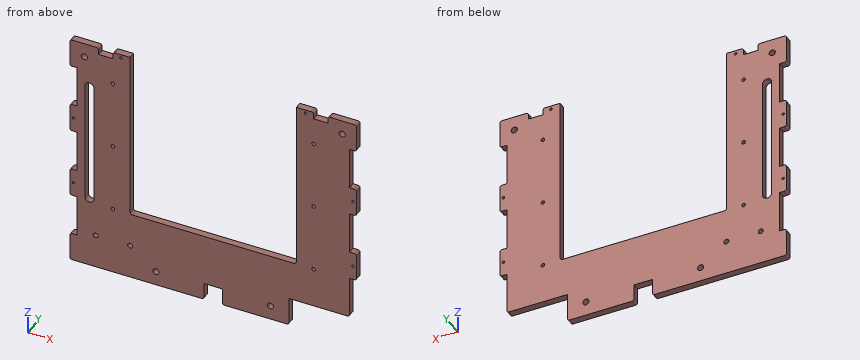
Autodesk Inventor part; units mm, degrees
ref_plane "YZ Plane" through (0, 0, 0) normal (1, 0, 0) x (0, 1, 0)
ref_plane "XZ Plane" through (0, 0, 0) normal (0, 1, 0) x (-1, 0, 0)
ref_plane "XY Plane" through (0, 0, 0) normal (0, 0, 1) x (1, 0, 0)
sketch "Sketch1" plane through (0, 0, 0) normal (0, 1, 0) x (-1, 0, 0)
  line L0 (125, -92.5) -> (-125, -92.5)
  line L1 (-125, -92.5) -> (-125, 92.5)
  line L2 (-125, 92.5) -> (125, 92.5)
  line L3 (125, 92.5) -> (125, -92.5)
  line L4 (125, -92.5) -> (-125, 92.5) construction
  line L5 (-125, -92.5) -> (125, 92.5) construction
  line L6 (72.5, -57.5) -> (-72.5, -57.5)
  line L7 (-72.5, -57.5) -> (-72.5, 57.5)
  line L8 (-72.5, 57.5) -> (72.5, 57.5)
  line L9 (72.5, 57.5) -> (72.5, -57.5)
  line L10 (72.5, -57.5) -> (-72.5, 57.5) construction
  line L11 (-72.5, -57.5) -> (72.5, 57.5) construction
  line L12 (-90.9745, -29.5734) -> (-84.0255, -29.5734) construction
  line L13 (-84.0255, -29.5734) -> (-84.0255, 29.5734) construction
  line L14 (-84.0255, 29.5734) -> (-90.9745, 29.5734) construction
  line L15 (-90.9745, 29.5734) -> (-90.9745, -29.5734) construction
  line L16 (-90.9745, -29.5734) -> (-84.0255, 29.5734) construction
  line L17 (-84.0255, -29.5734) -> (-90.9745, 29.5734) construction
  line L18 (81.5853, -29.5734) -> (93.4147, -29.5734) construction
  line L19 (93.4147, -29.5734) -> (93.4147, 29.5734) construction
  line L20 (93.4147, 29.5734) -> (81.5853, 29.5734) construction
  line L21 (81.5853, 29.5734) -> (81.5853, -29.5734) construction
  line L22 (81.5853, -29.5734) -> (93.4147, 29.5734) construction
  line L23 (93.4147, -29.5734) -> (81.5853, 29.5734) construction
  point P0 (0, 0)
  point P1 (-87.5, 0)
  point P2 (87.5, 0)
  dimension "d0" = 175
  dimension "d1" = 87.5
  dimension "d2" = 145
  dimension "d4" = 185
  dimension "d5" = 250
  dimension "d15" = 35
extrude "Extrusion1" add sketch "Sketch1" along normal blind 6
sketch "Sketch2" plane through (0, 6, 0) normal (0, 1, 0) x (1, 0, 0)
  line L0 (72.5, -57.5) -> (-72.5, -57.5)
  line L1 (-125, -92.5) -> (125, -92.5)
  line L2 (-72.5, -57.5) -> (72.5, -57.5)
  line L3 (72.5, -57.5) -> (72.5, -92.5)
  line L4 (72.5, -92.5) -> (-72.5, -92.5)
  line L5 (-72.5, -92.5) -> (-72.5, -57.5)
  point P0 (0, 0)
extrude "Extrusion2" cut sketch "Sketch2" against normal through all
sketch "Sketch3" plane through (0, 0, 0) normal (0, -1, 0) x (1, 0, 0)
  line L0 (-125, 92.5) -> (-125, -92.5)
  line L1 (-125, -92.5) -> (125, -92.5)
  line L2 (125, -92.5) -> (125, 92.5)
  line L3 (-125, -117.5) -> (66, -117.5)
  line L4 (66, -117.5) -> (66, -92.5)
  line L5 (66, -92.5) -> (-125, -92.5)
  line L6 (-125, -92.5) -> (-125, -117.5)
  line L7 (-125, -117.5) -> (66, -92.5) construction
  line L8 (66, -117.5) -> (-125, -92.5) construction
  point P0 (0, 0)
  point P1 (-29.5, -105)
  dimension "d10" = 59
  dimension "d11" = 25
extrude "Extrusion3" add sketch "Sketch3" against normal blind 6
sketch "Sketch4" plane through (0, 6, 0) normal (0, 1, 0) x (1, 0, 0)
  line L0 (-72.5, -92.5) -> (-72.5, 57.5)
  line L1 (-72.5, 57.5) -> (72.5, 57.5)
  line L2 (-125, -92.5) -> (-72.5, -92.5)
  line L3 (-108, 53.5) -> (-108, -52.5) construction
  line L4 (-112, 53.5) -> (-112, -52.5)
  line L5 (-104, -52.5) -> (-104, 53.5)
  arc A0 (-104, 53.5) -> (-112, 53.5) centre (-108, 53.5) ccw
  arc A1 (-112, -52.5) -> (-104, -52.5) centre (-108, -52.5) ccw
  point P0 (0, 0)
  point P1 (-108, 0.5)
  dimension "d16" = 8
  dimension "d17" = 108
  dimension "d18" = 40
extrude "Extrusion4" cut sketch "Sketch4" against normal through all
sketch "Sketch5" plane through (0, 0, 0) normal (0, -1, 0) x (1, 0, 0)
  line L0 (125, 92.5) -> (-125, 92.5)
  line L1 (72.5, -57.5) -> (-72.5, -57.5)
  circle A0 centre (-87.5, 62.5) radius 1.6
  circle A1 centre (-87.5, 2.5) radius 1.6
  circle A2 centre (-87.5, -57.5) radius 1.6
  circle A3 centre (87.5, 62.5) radius 1.6
  circle A4 centre (87.5, 2.5) radius 1.6
  circle A5 centre (87.5, -57.5) radius 1.6
  line L2 (87.5, 62.5) -> (-87.5, 62.5) construction
  line L3 (0, -57.5) -> (0, 62.5) construction
  line L4 (-95, -72.5) -> (-80, -72.5) construction
  line L5 (-80, -72.5) -> (-80, 77.5) construction
  line L6 (-80, 77.5) -> (-95, 77.5) construction
  line L7 (-95, 77.5) -> (-95, -72.5) construction
  line L8 (-95, -72.5) -> (-80, 77.5) construction
  line L9 (-80, -72.5) -> (-95, 77.5) construction
  point P0 (-72.5, 92.5)
  point P1 (0, 0)
  dimension "d21" = 60
  dimension "d22" = 60
  dimension "d23" = 175
  dimension "d24" = 3.2
  dimension "d25" = 150
  dimension "d26" = 15
extrude "Extrusion5" cut sketch "Sketch5" against normal through all
sketch "Sketch6" plane through (0, 6, 0) normal (0, 1, 0) x (1, 0, 0)
  circle A0 centre (-87.5, 57.5) radius 1.6
  line L0 (66, 117.5) -> (-125, 117.5)
  line L1 (-112.5, 60.5) -> (-62.5, 60.5) construction
  line L2 (-62.5, 60.5) -> (-62.5, 114.5) construction
  line L3 (-62.5, 114.5) -> (-112.5, 114.5) construction
  line L4 (-112.5, 114.5) -> (-112.5, 60.5) construction
  line L5 (-112.5, 60.5) -> (-62.5, 114.5) construction
  line L6 (-62.5, 60.5) -> (-112.5, 114.5) construction
  circle A1 centre (-102.5, 87.5) radius 2.2
  circle A2 centre (-72.5, 87.5) radius 2.2
  circle A3 centre (-50, 105) radius 2.7
  circle A4 centre (50, 105) radius 2.7
  line L7 (125, -92.5) -> (125, 92.5)
  line L8 (-125, 117.5) -> (-125, -92.5)
  line L9 (-125, -92.5) -> (-72.5, -92.5)
  circle A5 centre (-112.5, -80) radius 2.7
  circle A6 centre (112.5, -80) radius 2.7
  point P0 (0, 0)
  point P1 (-87.5, 87.5)
  dimension "d29" = 50
  dimension "d30" = 54
  dimension "d31" = 3
  dimension "d32" = 4.4
  dimension "d33" = 30
  dimension "d34" = 15
  dimension "d42" = 12.5
  dimension "d43" = 50
  dimension "d44" = 50
  dimension "d45" = 5.4
  dimension "d46" = 12.5
  dimension "d47" = 12.5
  dimension "d48" = 12.5
  dimension "d49" = 5.4
  dimension "d71" = 12.5
extrude "Extrusion6" cut sketch "Sketch6" against normal through all contours A1 | A2 | A3 | A4 | A5 | A6
sketch "Sketch7" plane through (0, 6, 0) normal (0, 1, 0) x (1, 0, 0)
  line L0 (66, 117.5) -> (-125, 117.5)
  line L1 (-8, 102.5) -> (8, 102.5)
  line L2 (8, 102.5) -> (8, 117.5)
  line L3 (8, 117.5) -> (-8, 117.5)
  line L4 (-8, 117.5) -> (-8, 102.5)
  line L5 (-8, 102.5) -> (8, 117.5) construction
  line L6 (8, 102.5) -> (-8, 117.5) construction
  point P0 (0, 0)
  point P1 (0, 110)
  dimension "d38" = 16
  dimension "d39" = 15
extrude "Extrusion7" cut sketch "Sketch7" against normal through all
sketch "Sketch8" plane through (0, 6, 0) normal (0, 1, 0) x (1, 0, 0)
  line L0 (-125, 117.5) -> (-125, -92.5)
  line L1 (72.5, -92.5) -> (125, -92.5)
  line L2 (125, -92.5) -> (125, 92.5)
  line L3 (125, 92.5) -> (66, 92.5)
  line L4 (125, 92.5) -> (118.9, 92.5)
  line L5 (118.9, 92.5) -> (118.9, 55.8333)
  line L6 (118.9, 55.8333) -> (125, 55.8333)
  line L7 (125, 55.8333) -> (125, 92.5)
  line L8 (125, -67.5) -> (118.9, -67.5)
  line L9 (118.9, -67.5) -> (118.9, -30.8333)
  line L10 (118.9, -30.8333) -> (125, -30.8333)
  line L11 (125, -30.8333) -> (125, -67.5)
  line L12 (125, 30.8333) -> (118.9, 30.8333)
  line L13 (118.9, 30.8333) -> (118.9, -5.8333)
  line L14 (118.9, -5.8333) -> (125, -5.8333)
  line L15 (125, -5.8333) -> (125, 30.8333)
  line L16 (-125, 92.5) -> (-118.9, 92.5)
  line L17 (-118.9, 92.5) -> (-118.9, 55.8333)
  line L18 (-118.9, 55.8333) -> (-125, 55.8333)
  line L19 (-125, 55.8333) -> (-125, 92.5)
  line L20 (-125, 30.8333) -> (-118.9, 30.8333)
  line L21 (-118.9, 30.8333) -> (-118.9, -5.8333)
  line L22 (-118.9, -5.8333) -> (-125, -5.8333)
  line L23 (-125, -5.8333) -> (-125, 30.8333)
  line L24 (-125, -67.5) -> (-118.9, -67.5)
  line L25 (-118.9, -67.5) -> (-118.9, -30.8333)
  line L26 (-118.9, -30.8333) -> (-125, -30.8333)
  line L27 (-125, -30.8333) -> (-125, -67.5)
  circle A0 centre (121.95, 43.3333) radius 1.1
  circle A1 centre (121.95, -18.3333) radius 1.1
  circle A2 centre (-121.95, -18.3333) radius 1.1
  circle A3 centre (-121.95, 43.3333) radius 1.1
  line L28 (121.95, 55.8333) -> (121.95, 43.3333) construction
  line L29 (-121.95, 55.8333) -> (-121.95, 43.3333) construction
  point P0 (0, 0)
  dimension "d50" = 25
  dimension "d51" = 6.1
  dimension "d52" = 25
  dimension "d53" = 25
  dimension "d54" = 2.2
  dimension "d55" = 12.5
  dimension "d56" = 12.5
extrude "Extrusion8" cut sketch "Sketch8" against normal through all
sketch "Sketch9" plane through (0, 6, 0) normal (0, 1, 0) x (1, 0, 0)
  circle A0 centre (-121.95, -18.3333) radius 1.1
  line L0 (-118.9, -67.5) -> (-125, -67.5)
  line L1 (-125, -92.5) -> (-72.5, -92.5)
  line L2 (72.5, -92.5) -> (125, -92.5)
  line L3 (-100, -92.5) -> (-87.5, -92.5)
  line L4 (-87.5, -92.5) -> (-87.5, -86.4)
  line L5 (-87.5, -86.4) -> (-100, -86.4)
  line L6 (-100, -86.4) -> (-100, -92.5)
  line L7 (100, -92.5) -> (87.5, -92.5)
  line L8 (87.5, -92.5) -> (87.5, -86.4)
  line L9 (87.5, -86.4) -> (100, -86.4)
  line L10 (100, -86.4) -> (100, -92.5)
  circle A1 centre (-80.5, -89.45) radius 1.1
  circle A2 centre (80.5, -89.45) radius 1.1
  line L11 (-80.5, -89.45) -> (-87.5, -89.45) construction
  line L12 (-125, -67.5) -> (-125, -92.5)
  line L13 (-72.5, -92.5) -> (-72.5, 57.5)
  line L14 (72.5, 57.5) -> (72.5, -92.5)
  line L15 (125, -92.5) -> (125, -67.5)
  point P0 (0, 0)
  dimension "d60" = 12.5
  dimension "d66" = 25
  dimension "d68" = 8
  dimension "d69" = 8
  dimension "d70" = 25
extrude "Extrusion9" cut sketch "Sketch9" against normal through all contours L6 L5 L4 L1 | L8 L9 L10 L2 | A1 | A2
fillet "Fillet1" radius 2 9 edges at (125, 3, 92.5) (72.5, 3, -57.5) (-125, 3, 92.5) (-72.5, 3, -57.5) (66, 3, -117.5) (-125, 3, -117.5) (8, 3, -117.5) (-8, 3, -117.5) (118.9, 3, -92.5)
fillet "Fillet2" radius 2 15 edges at (125, 3, -55.8333) (125, 3, -30.8333) (125, 3, 5.8333) (125, 3, 30.8333) (125, 3, 67.5) (-125, 3, 67.5) (-125, 3, 30.8333) (-125, 3, 5.8333) (-125, 3, -30.8333) (-125, 3, -55.8333) (-125, 3, -92.5) (-100, 3, 92.5) (-87.5, 3, 92.5) (87.5, 3, 92.5) (100, 3, 92.5)
equation "\"d22\" = d21"
equation "\"d53\" = d52"
equation "\"d55\" = 0.5 * d52"
equation "\"d56\" = d55"
properties part number "InnerTop"
Model file for the job. Use its own axes, mm. Round coordinates to 2 decimals unless told otherwise and drop trailing zeros. Order: outer loops, then holes, each group sorted by start corner. A loop starts at its lowest first (then second) coordinate and runs counter-clockwise, first axis right, second up. Notation, with made-up numbers: (56, -5) -> (91, -5) arc R9 cw to (91, -1) -> close; hole circle Ø2 at (-3.5, 5.5). An arc over 180 degrees is marked (long way). Use one line per item in the form item = value.
Item 1: Cut at D-D, the plane y = 5.05. Give the number of separate pieces and of enclosed holes in the cut face, and give its area (3 significant figures).
Returned:
separate_pieces = 1
enclosed_holes = 19
area = 26,400 mm^2
Item 2: Cut at A-A, the plane z = -50. Write the cut outline in (x, y), and give its area (3 significant figures).
Returned:
outline = (-125, 0) -> (-112, 0) -> (-112, 6) -> (-125, 6) -> close; (-104, 0) -> (-72.5, 0) -> (-72.5, 6) -> (-104, 6) -> close; (72.5, 0) -> (125, 0) -> (125, 6) -> (72.5, 6) -> close
area = 582 mm^2
Item 3: Cut at C-C, the plane z = 47. Write the cut outline in (x, y).
Returned:
outline = (-118.9, 0) -> (-112, 0) -> (-112, 6) -> (-118.9, 6) -> close; (-104, 0) -> (-72.5, 0) -> (-72.5, 6) -> (-104, 6) -> close; (72.5, 0) -> (118.9, 0) -> (118.9, 6) -> (72.5, 6) -> close
Item 4: Cut at B-B, the plane x = 50. Write the cut outline in (y, z), and give its area (3 significant figures).
Returned:
outline = (0, -117.5) -> (6, -117.5) -> (6, -107.7) -> (0, -107.7) -> close; (0, -102.3) -> (6, -102.3) -> (6, -57.5) -> (0, -57.5) -> close
area = 328 mm^2
Item 5: Drill centre lines: line 1 (X direction, y = 4.6, z = 80); line 2 (X direction, y = 1.9, z = -14); line 3 (X direction, y = 4.4, z = 12). Where is each one in solid material? Low to high.
Returned:
line_1 = -125 to -115.2, -109.8 to -72.5, 72.5 to 109.8, 115.2 to 125
line_2 = -118.9 to -112, -104 to -72.5, 72.5 to 118.9
line_3 = -125 to -112, -104 to -72.5, 72.5 to 125
Item 6: Flat gauge pins, fed straight in: pin 1 Ø8.5 at (x, z) = (-112.5, 80) entering from +Y; pin 2 Ø2 at (x, z) = (121.95, -43.33) entering from +Y; pin 3 Ø1 at (x, y) = (-88.5, 3) entering from +Z; pin 4 Ø3 at (x, y) = (93.5, 4) entering from -Z. Where does each tip first touch, or does it go through?
Returned:
pin_1 = 6
pin_2 = through
pin_3 = 86.4
pin_4 = -92.5
